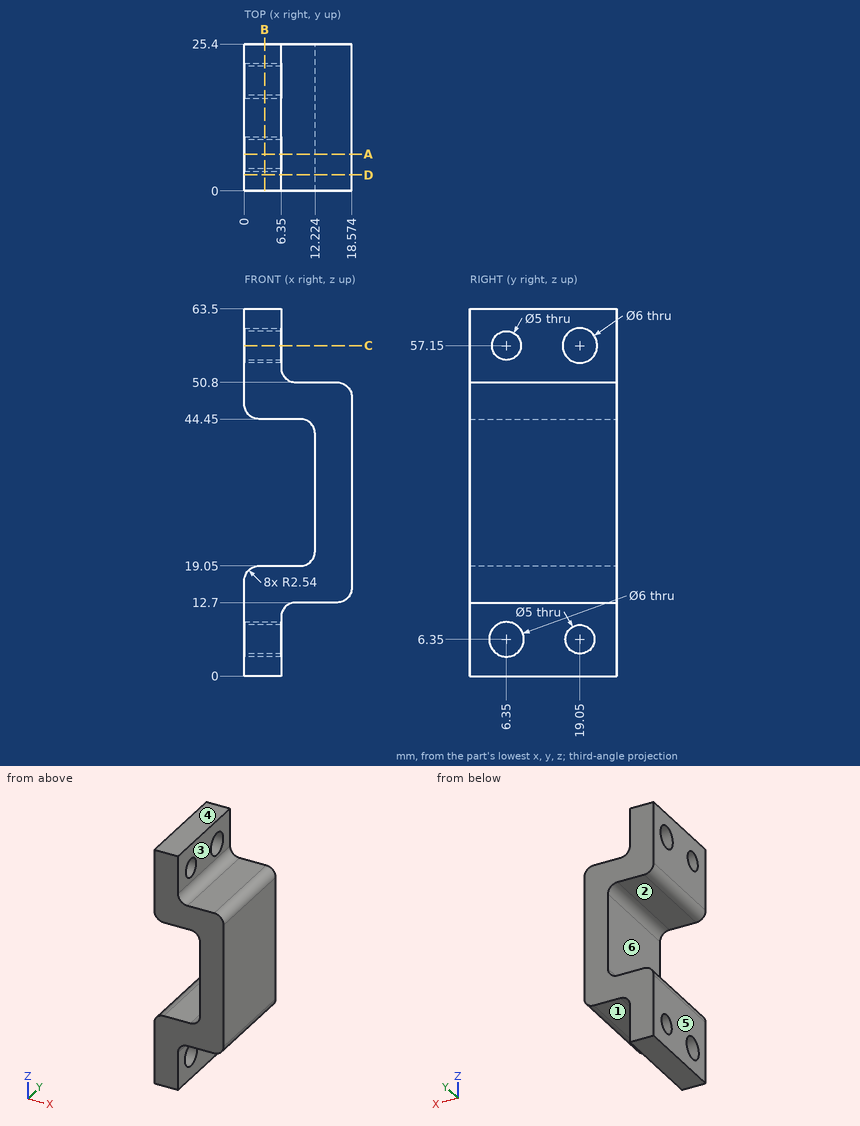
Design review of the part shown in the three views and the two pictorial views. Dimensions are in mm from the part's minimum x, y and z. A direction names the side the tool comes from. Coordinates: 2 decimals unless noted, no trailing zeros. Write each loop counter-clockwise with the first axis right and the second up, starting at its lowest first coordinate (ties: lowest second). Pieces come first, ordered by that corner, then holes. Notation, with made-up numbers: (0.5, -38.5) -> (28.5, -38.5) arc R4 cw to (28.5, -34.5) -> close; hole circle Ø2 at (5.5, 70). An arc over 180 degrees is marked (long way). Answer in a Markdown table with one row per item.
1. We need section D-D, the plane y = 2.75. State the section outline as (x, z) points.
Answers below:
| item | result |
|---|---|
| outline | (0, 0) -> (6.35, 0) -> (6.35, 10.16) arc R2.54 cw to (8.89, 12.7) -> (16.03, 12.7) arc R2.54 ccw to (18.57, 15.24) -> (18.57, 48.26) arc R2.54 ccw to (16.03, 50.8) -> (8.89, 50.8) arc R2.54 cw to (6.35, 53.34) -> (6.35, 63.5) -> (0, 63.5) -> (0, 46.99) arc R2.54 ccw to (2.54, 44.45) -> (9.68, 44.45) arc R2.54 cw to (12.22, 41.91) -> (12.22, 21.59) arc R2.54 cw to (9.68, 19.05) -> (2.54, 19.05) arc R2.54 ccw to (0, 16.51) -> close |
2. Draft analysis for pull direction Z (two halves, no side actions). For the marked faces 4, 5 and 6, state which applies: +Z half, -Z half, draft (parallel to the pull), parting line (faces both ways), or undercut.
Answers below:
| item | result |
|---|---|
| face 4 | +Z half |
| face 5 | draft |
| face 6 | undercut |
3. We need section A-A, the plane y = 6.35. State the section outline as (x, z) points.
Answers below:
| item | result |
|---|---|
| outline | (0, 0) -> (6.35, 0) -> (6.35, 3.35) -> (0, 3.35) -> close; (0, 9.35) -> (6.35, 9.35) -> (6.35, 10.16) arc R2.54 cw to (8.89, 12.7) -> (16.03, 12.7) arc R2.54 ccw to (18.57, 15.24) -> (18.57, 48.26) arc R2.54 ccw to (16.03, 50.8) -> (8.89, 50.8) arc R2.54 cw to (6.35, 53.34) -> (6.35, 54.65) -> (0, 54.65) -> (0, 46.99) arc R2.54 ccw to (2.54, 44.45) -> (9.68, 44.45) arc R2.54 cw to (12.22, 41.91) -> (12.22, 21.59) arc R2.54 cw to (9.68, 19.05) -> (2.54, 19.05) arc R2.54 ccw to (0, 16.51) -> close; (0, 59.65) -> (6.35, 59.65) -> (6.35, 63.5) -> (0, 63.5) -> close |
4. We need section B-B, the plane x = 3.5. State the section outline as (y, z) points, and give its area (3 significant figures).
Answers below:
| item | result |
|---|---|
| outline | (0, 0) -> (25.4, 0) -> (25.4, 19.05) -> (0, 19.05) -> close; (0, 44.45) -> (25.4, 44.45) -> (25.4, 63.5) -> (0, 63.5) -> close; hole circle Ø6 at (6.35, 6.35); hole circle Ø5 at (6.35, 57.15); hole circle Ø6 at (19.05, 57.15); hole circle Ø5 at (19.05, 6.35) |
| area | 872 mm^2 |
5. We need section C-C, the plane z = 57.15. State the section outline as (x, y) points.
Answers below:
| item | result |
|---|---|
| outline | (0, 0) -> (6.35, 0) -> (6.35, 3.85) -> (0, 3.85) -> close; (0, 8.85) -> (6.35, 8.85) -> (6.35, 16.05) -> (0, 16.05) -> close; (0, 22.05) -> (6.35, 22.05) -> (6.35, 25.4) -> (0, 25.4) -> close |
6. Clearance check with flat-ended pins moving along their axes: pin 1 Ø4 at (x, y) = (15.5, 7.5) entering from +Z; pin 2 Ø8 at (x, y) = (13, 11.5) entering from -Z; pin 3 Ø3 at (x, y) = (3.5, 4) entering from -Z; pin 4 Ø4 at (y, z) = (10.5, 32.5) entering from -X. State where each tip first meets the part, or that it passes through.
Answers below:
| item | result |
|---|---|
| pin 1 | stops at z = 50.8 |
| pin 2 | stops at z = 12.7 |
| pin 3 | stops at z = 0 |
| pin 4 | stops at x = 12.22 |
7. Wall thickness on probe 1 along Y at (x, z) = (3.5, 57.15); probe 2 along Y at (x, z) = (2.5, 6.35); probe 3 along X at (y, z) = (21.5, 29): over which ranges is each line inside the solid? List them lowest first. Write a range as [from, to].
Answers below:
| item | result |
|---|---|
| probe 1 | y = [0, 3.85], [8.85, 16.05], [22.05, 25.4] |
| probe 2 | y = [0, 3.35], [9.35, 16.55], [21.55, 25.4] |
| probe 3 | x = [12.22, 18.57] |
8. For the marked faces 1, 2 and 3, list the 3-axis set-ups (+Z, -Z, +X, -X, +Y, -Y) from which the entire face can be reached by the end or side of a thin tool; tool diameter is ignored.
Answers below:
| item | result |
|---|---|
| face 1 | -Z, +X, +Y, -Y |
| face 2 | -X, +Y, -Y |
| face 3 | +Z, +X, +Y, -Y |
